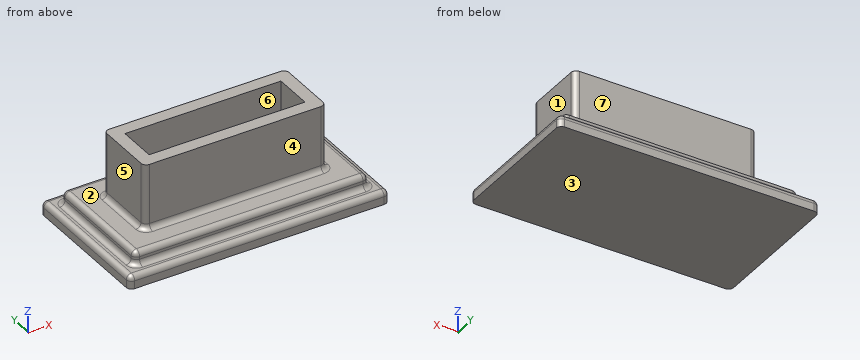
from build123d import *

# Parameters (mm, degrees)
F0_W     = 100
F0_H     = 54.953308776
F1_DEPTH = 5
F2_W     = 90
F2_H     = 44.953308776
F3_DEPTH = 5
F4_W     = 70
F4_H     = 24.953308776
F5_DEPTH = 25
F6_R     = 2
F7_W     = 60
F7_H     = 14.953308776
F8_DEPTH = 25


with BuildPart() as f1:
    # F0 (on Top) → F1 (new body)
    with BuildSketch(Plane.XY):
        with Locations((10.9343037009, -2.2429926321)):
            Rectangle(F0_W, F0_H)
    extrude(amount=F1_DEPTH)

    # F2 (on face) → F3 (join)
    with BuildSketch(Plane.XY.offset(5)):
        with Locations((10.9343037009, -2.2429926321)):
            Rectangle(F2_W, F2_H)
    extrude(amount=F3_DEPTH)

    # F4 (on face) → F5 (join)
    with BuildSketch(Plane.XY.offset(10)):
        with Locations((10.9343037009, -2.2429926321)):
            Rectangle(F4_W, F4_H)
    extrude(amount=F5_DEPTH)

    # F6
    f6_edges = [f1.edges().sort_by_distance(p)[0] for p in [
        (60.934304, 25.233662, 2.5),
        (-39.065696, 25.233662, 2.5),
        (-39.065696, -29.719647, 2.5),
        (60.934304, -29.719647, 2.5),
        (45.934304, -14.719647, 22.5),
        (45.934304, 10.233662, 22.5),
        (55.934304, 20.233662, 7.5),
        (55.934304, -24.719647, 7.5),
        (-24.065696, -14.719647, 22.5),
        (-24.065696, 10.233662, 22.5),
        (-34.065696, -24.719647, 7.5),
        (-34.065696, 20.233662, 7.5),
        (10.934304, -24.719647, 5),
        (10.934304, -14.719647, 10),
        (10.934304, -24.719647, 10),
        (10.934304, -29.719647, 5),
        (60.934304, -2.242993, 5),
        (10.934304, 25.233662, 5),
        (-39.065696, -2.242993, 5),
        (55.934304, -2.242993, 5),
        (10.934304, 20.233662, 5),
        (-34.065696, -2.242993, 5),
        (45.934304, -2.242993, 10),
        (-34.065696, -2.242993, 10),
        (55.934304, -2.242993, 10),
        (10.934304, 20.233662, 10),
        (10.934304, 10.233662, 10),
        (-24.065696, -2.242993, 10),
    ]]
    fillet(f6_edges, radius=F6_R)

    # F7 (on face) → F8 (cut)
    with BuildSketch(Plane.XY.offset(35)):
        with Locations((10.9343037009, -2.2429926321)):
            Rectangle(F7_W, F7_H)
    extrude(amount=-F8_DEPTH, mode=Mode.SUBTRACT)


solid = f1.part
The model under review builds one solid part; all positions refer to its coordinate system, in mm. Face numbers are marked on the shaded views. A direction names the side the tool comes from. Give positions to 0.01 mm unless a question says otherwise; leave off trailing zeros. Loops run counter-clockwise (first coordinate to the right, second up) from the corner with the lowest first, then second, coordinate; pieces in that order, holes last. Notation, with made-up numbers: (-13, -19) -> (27, -19) arc R10 cw to (27, -5) -> close; hole circle Ø7 at (44.5, 47). An arc over 180 degrees is marked (long way). Answer as a JSON object with one key per item and string values. Group by question number.
Q1. Take a section at C-C (y = -11). Write out the cut boundary in (x, z).
Q2. Take a section at D-D (z = 11). Write out the cut boundary in (x, y), plus the area to 3 significant figures.
Q3. Take a section at B-B (x = 27.5). Write out the cut boundary in (y, z), plus the area to 3 significant figures.
Q4. Draft analysis for pull direction Y (two halves, no side actions). For the marked faces 4, 5, 6 and 7, state which applies: pulls with the +Y half, pulls with the -Y half, needs draft (parallel to the pull), parting line crosses it, or undercut.
Q5. Wall thickness on line 1 along Y through (x, z) = (0, 25); line 2 along X through (y, z) = (-9.5, 19.5); line 3 along Z through (x, y) = (20, 22.5): over which ranges is each line inside the solid? List them lowest first.
Q6. Take a section at A-A (z = 30.5). Write out the cut boundary in (x, y), plus the area to 3 significant figures.
Q7. Insertion check: pin 1 (1.1 mm diameter, centred on x = 14.5, z = 7.5, fed in from +Y); pin 2 (2 mm diameter, centred on x = 22, y = -3.5, fed in from +Z); pin 3 (7.5 mm diameter, centred on x = 17.5, z = 25, fed in from +Y); pin 4 (5 mm diameter, centred on y = 13.5, z = 27, fed in from -X). Each pin has a flat end and moves straight along its axis. Give the tip position at first contact, or say it passes through.
Q8. Tool access review of the marked faces 1, 2 and 3: name each direction out of +Z, -Z, +X, -X, +Y, -Y from which nothing blocks a thin tool from reaching the whole face with its end or side.
Answer below:
{
 "1": {"outline": "(-39.07, 0) -> (60.93, 0) -> (60.93, 3) arc R2 ccw to (58.93, 5) -> (57.93, 5) arc R2 cw to (55.93, 7) -> (55.93, 8) arc R2 ccw to (53.93, 10) -> (47.93, 10) arc R2 cw to (45.93, 12) -> (45.93, 35) -> (-24.07, 35) -> (-24.07, 12) arc R2 cw to (-26.07, 10) -> (-32.07, 10) arc R2 ccw to (-34.07, 8) -> (-34.07, 7) arc R2 cw to (-36.07, 5) -> (-37.07, 5) arc R2 ccw to (-39.07, 3) -> close"},
 "2": {"outline": "(-24.33, -12.72) arc R2.27 ccw to (-22.07, -14.99) -> (43.93, -14.99) arc R2.27 ccw to (46.2, -12.72) -> (46.2, 8.23) arc R2.27 ccw to (43.93, 10.5) -> (-22.07, 10.5) arc R2.27 ccw to (-24.33, 8.23) -> close; hole (-19.07, -9.72) -> (40.93, -9.72) -> (40.93, 5.23) -> (-19.07, 5.23) -> close", "area": "896 mm2"},
 "3": {"outline": "(-29.72, 0) -> (25.23, 0) -> (25.23, 3) arc R2 ccw to (23.23, 5) -> (22.23, 5) arc R2 cw to (20.23, 7) -> (20.23, 8) arc R2 ccw to (18.23, 10) -> (12.23, 10) arc R2 cw to (10.23, 12) -> (10.23, 35) -> (5.23, 35) -> (5.23, 10) -> (-9.72, 10) -> (-9.72, 35) -> (-14.72, 35) -> (-14.72, 12) arc R2 cw to (-16.72, 10) -> (-22.72, 10) arc R2 ccw to (-24.72, 8) -> (-24.72, 7) arc R2 cw to (-26.72, 5) -> (-27.72, 5) arc R2 ccw to (-29.72, 3) -> close", "area": "750 mm2"},
 "4": {"face 4": "pulls with the -Y half", "face 5": "needs draft", "face 6": "undercut", "face 7": "pulls with the +Y half"},
 "5": {"line 1": "y = -14.72 to -9.72, 5.23 to 10.23", "line 2": "x = -24.07 to -19.07, 40.93 to 45.93", "line 3": "z = 0 to 5"},
 "6": {"outline": "(-24.07, -12.72) arc R2 ccw to (-22.07, -14.72) -> (43.93, -14.72) arc R2 ccw to (45.93, -12.72) -> (45.93, 8.23) arc R2 ccw to (43.93, 10.23) -> (-22.07, 10.23) arc R2 ccw to (-24.07, 8.23) -> close; hole (-19.07, -9.72) -> (40.93, -9.72) -> (40.93, 5.23) -> (-19.07, 5.23) -> close", "area": "846 mm2"},
 "7": {"pin 1": "stops at y = 20.23", "pin 2": "stops at z = 10", "pin 3": "stops at y = 10.23", "pin 4": "passes through"},
 "8": {"face 1": "+Z, +X, +Y, -Y", "face 2": "+Z", "face 3": "-Z, +X, -X, +Y, -Y"}
}
